Geometry: final body of the model. Coordinates: model frame, mm. A direction names the side the tool comes from. Give positions to 0.01 mm unless a question says otherwise; leave off trailing zeros. Write each loop counter-clockwise with the first axis right and the second up, starting at its lowest first coordinate (ties: lowest second). Pieces come first, ordered by that corner, then holes. Notation, with made-up numbers: M 8,34.5 L 64,34.5 A23 ccw 64,62.5 Z; hole C -27,53 d9. An arc over 180 degrees is marked long. Use a Markdown table: item, result. Add a question column.
1) Section A-A on x = 0. Return the cut outline in (y, z), then the cut area to 3 significant figures.
2) Set-up query: faces 1 (the flat face through (4.2, -1.7, 6.45)), 2 (the flat face through (-4.2, -1.7, 6.45)), 3 (the cylindrical face through (2.23, -1.15, 5.92)). Return all of +Z, -Z, +X, -X, +Y, -Y with unobstructed straight access to the full face (end or side cutting, diameter ignored); none if empty.
3) Section C-C on z = 3.5. Return the cut outline in (x, y).
4) Section B-B on z = 8. Return the cut outline in (x, y).
5) Draft query along Z for faces 4 (the flat face through (4.2, -1.7, 10.55)), 5 (the cylindrical face through (-2.27, -1.15, 5.92)), 6 (the flat face through (0, -1, 12)). Return one class per face: +Z half, -Z half, draft (parallel to the pull), parting line (faces both ways), or undercut.
6) Line query: line 1 (X direction, y = -1.25, z = 8); line 2 (Z direction, x = 0, y = -0.65); line 3 (X direction, y = -1.45, z = 10). Output: solid intervals per line, ascending.
7) Section D-D on y = -0.8. Return the cut outline in (x, z), then the cut area to 3 significant figures.
Autodesk Inventor part; units mm, degrees
ref_plane "Work Plane1" through (0, 0, 10.55) normal (0, 0, 1) x (1, 0, 0)
ref_plane "YZ Plane" through (0, 0, 0) normal (1, 0, 0) x (0, 1, 0)
ref_plane "XZ Plane" through (0, 0, 0) normal (0, 1, 0) x (-1, 0, 0)
sketch "Sketch1" plane through (0, 0, 0) normal (0, 0, 1) x (1, 0, 0)
  line L0 (-4.752, -2.1513) -> (-3.25, -2.1513)
  arc A0 (-1.25, -2.1513) -> (-3.25, -2.1513) centre (-2.25, -2.1513) ccw
  line L1 (-3.25, -2.1513) -> (1.2966, -2.1513) construction
  line L2 (-1.25, -2.1513) -> (1.25, -2.1513)
  arc A1 (3.25, -2.1513) -> (1.25, -2.1513) centre (2.25, -2.1513) ccw
  line L3 (1.25, -2.1513) -> (6.8796, -2.1513) construction
  line L4 (3.25, -2.1513) -> (4.752, -2.1513)
  line L5 (-4.752, -2.1513) -> (-3.886, -0.6513)
  line L6 (-4.752, -2.1513) -> (-3.02, -2.1513) construction
  arc A2 (-3.02, -0.1513) -> (-3.886, -0.6513) centre (-3.02, -1.1513) ccw
  line L7 (-3.886, -0.6513) -> (-3.02, -0.1513) construction
  line L8 (-3.02, -0.1513) -> (3.02, -0.1513)
  line L9 (4.752, -2.1513) -> (3.886, -0.6513)
  line L10 (4.752, -2.1513) -> (6.484, -2.1513) construction
  arc A3 (3.886, -0.6513) -> (3.02, -0.1513) centre (3.02, -1.1513) ccw
  line L11 (0, 0) -> (0, 1.588) construction
  dimension "d1" = 2
  dimension "d2" = 2.5
  dimension "d3" = 2
  dimension "d5" = 60
  dimension "d6" = 1.732
  dimension "d7" = 1
  dimension "d8" = 1
  dimension "d9" = 6.04
  dimension "d10" = 1.732
  dimension "d11" = 120
  dimension "d12" = 1
  dimension "d34" = 9.504
  dimension "d35" = 1.502
  dimension "d36" = 1.502
extrude "Extrusion1" add sketch "Sketch1" along normal blind 12
sketch "Sketch2" plane through (-3.02, -0.1513, 0) normal (0, 1, 0) x (1, 0, 0)
  line L0 (6.04, -12) -> (0, -12)
  line L1 (7.772, 0) -> (7.772, -12)
  point P0 (3.02, 0)
  point P1 (3.02, -8)
  dimension "d22" = 4
  dimension "d23" = 4.752
hole "Hole1" at (0, -0.1513, 8) direction (0, -1, 0) diameter 1.5 depth 8 tip angle 118
ref_plane "Work Plane1" through (0, 0, 10.55) normal (0, 0, 1) x (1, 0, 0)
sketch "Sketch3" plane through (0, 0, 10.55) normal (0, 0, 1) x (1, 0, 0)
  line L0 (-4.1458, -1.1013) -> (-3.9448, -1.1013)
  line L1 (-4.752, -2.1513) -> (-3.25, -2.1513)
  line L2 (-3.886, -0.6513) -> (-4.752, -2.1513)
  line L3 (-3.9448, -1.1013) -> (-3.6515, -1.5013)
  line L4 (-3.6515, -1.5013) -> (-4.0005, -1.5013)
  line L5 (-4.0005, -1.5013) -> (-4.0005, -1.8513)
  line L6 (-4.0005, -1.8513) -> (-3.8913, -2.1513)
  line L7 (-4.1458, -1.1013) -> (-4.752, -2.1513)
  line L8 (-4.752, -2.1513) -> (-3.8913, -2.1513)
  point P0 (0, 0)
  dimension "d25" = 1.05
  dimension "d26" = 0.201
  dimension "d27" = 126.25
  dimension "d28" = 0.496
  dimension "d29" = 0.349
  dimension "d30" = 0.35
  dimension "d31" = 160
extrude "Extrusion2" cut sketch "Sketch3" against normal blind 4.1
mirror "Mirror1" about plane through (0, 0, 0) normal (1, 0, 0) of "Extrusion2"
properties part number "3d_LM - Pinza 1" material "PA12 SLS 3D Print"
Found:
| question | item | result |
|---|---|---|
| 1 | outline | M -2.15,0 L -0.15,0 L -0.15,7.25 L -2.15,7.25 Z; M -2.15,8.75 L -0.15,8.75 L -0.15,12 L -2.15,12 Z |
| 1 | area | 21.0 mm² |
| 2 | face 1 | +X |
| 2 | face 2 | -X |
| 2 | face 3 | +Z, -Z, -Y |
| 3 | outline | M -4.75,-2.15 L -3.25,-2.15 A1 cw -1.25,-2.15 L 1.25,-2.15 A1 cw 3.25,-2.15 L 4.75,-2.15 L 3.89,-0.65 A1 ccw 3.02,-0.15 L -3.02,-0.15 A1 ccw -3.89,-0.65 Z |
| 4 | outline | M -4.15,-1.1 L -3.94,-1.1 L -3.65,-1.5 L -4,-1.5 L -4,-1.85 L -3.89,-2.15 L -3.25,-2.15 A1 cw -1.25,-2.15 L -0.75,-2.15 L -0.75,-0.15 L -3.02,-0.15 A1 ccw -3.89,-0.65 Z; M 0.75,-2.15 L 1.25,-2.15 A1 cw 3.25,-2.15 L 3.89,-2.15 L 4,-1.85 L 4,-1.5 L 3.65,-1.5 L 3.94,-1.1 L 4.15,-1.1 L 3.89,-0.65 A1 ccw 3.02,-0.15 L 0.75,-0.15 Z |
| 5 | face 4 | undercut |
| 5 | face 5 | draft |
| 5 | face 6 | +Z half |
| 6 | line 1 | -3.84 to -2.68, -1.82 to -0.75, 0.75 to 1.82, 2.68 to 3.84 |
| 6 | line 2 | 0 to 7.25, 8.75 to 12 |
| 6 | line 3 | -3.69 to -2.96, -1.54 to 1.54, 2.96 to 3.69 |
| 7 | outline | M -3.97,0 L 3.97,0 L 3.97,12 L -3.97,12 Z; hole C 0,8 d1.5 |
| 7 | area | 93.6 mm² |
